Geometry: final body of the model. Coordinates: model frame, mm. A direction names the side the tool comes from. Give positions to 0.01 mm unless a question says otherwise; leave off trailing zeros. Write each loop counter-clockwise with the first axis right and the second up, starting at its lowest first coordinate (ties: lowest second). Pieces come first, ordered by that corner, then holes.
Q1. Cut plane A-A on x = -11.65. Return the cut outline in (y, z).
Q2. Line query: L1, parallel to X at y = 2.5, z = -10.5; L2, parallel to X at y = 0.5, z = -11.85; L3, parallel to X at y = 0.85, z = -11.85. Output: solid intervals per line, ascending.
Q3. Cut plane B-B on z = 4. Return the cut outline in (x, y).
Q4. Pin query (flat end, axial travel): pin 1 (1 mm diameter, centred on y = 7, z = -10.5, fed in from +X); pin 2 (0.6 mm diameter, centred on y = 1.5, z = 1.5, fed in from -X); pin 3 (3.5 mm diameter, centred on y = 7, z = 2.5, fed in from -X); pin 4 (2.5 mm diameter, centred on x = -11.65, z = -11.85, fed in from +Y) (3 decimals). Return the tip coordinate at first contact, or that it passes through.
Q5. Cut plane C-C on x = 8.5. Return the cut outline in (y, z).
Q6. Draft query along Z for faces 1 (the face through (-10.15, 0.99, -11.92)), 2 (the face through (19.213, 0.986, -19.353)), 3 (the face through (19.37, 1.01, 19.23)). Return one class per face: pulls with the +Z half, pulls with the -Z half, needs draft (parallel to the pull), parting line crosses it, or undercut.
Q7. Cut plane D-D on z = 11.85. Return the cut outline in (x, y).
Q8. Reachability of faces 4 (the face through (13.136, 6, 21)), 5 (the face through (0, 1, -9.75)), 6 (the face through (0, 4, 14)) from +Z, -Z, +X, -X, +Y, -Y: full face, straight path, thin tool, end or side. Return the list, or none.
```python
from build123d import *

# Parameters (mm, degrees)
BOSS_EXTRUDE1_DEPTH = 5
BOSS_EXTRUDE2_DEPTH = 3
CHAMFER1_SIZE       = 2
SKETCH4_R           = 1.5
SKETCH4_W           = 27.5
SKETCH4_H           = 19.5
CUT_EXTRUDE2_DEPTH  = 8
SKETCH5_W           = 28
SKETCH5_H           = 28
CUT_EXTRUDE3_DEPTH  = 3


with BuildPart() as part:
    # Sketch1 → Boss-Extrude1 (new body)
    with BuildSketch(Plane(origin=(0, 0, 0), x_dir=(1, 0, 0), z_dir=(0, 1, 0))):
        Polygon((15, 25), (25, 15), (25, -15), (15, -25), (-25, -25), (-25, 25), align=None)
    extrude(amount=BOSS_EXTRUDE1_DEPTH)

    # Sketch2 → Boss-Extrude2 (add)
    with BuildSketch(Plane(origin=(0, 5, 0), x_dir=(1, 0, 0), z_dir=(0, 1, 0))):
        Polygon((-20.5, 20.5), (-20.5, -20.5), (-22.5, -22.5), (-22.5, 22.5), align=None)
        Polygon((13.964466094, 22.5), (13.136038969, 22.5), (13.136038969, 20.5), (20.5, 13.136038969), (22.5, 13.136038969), (22.5, 13.964466094), align=None)
        Polygon((13.136038969, -20.5), (13.136038969, -22.5), (13.964466094, -22.5), (22.5, -13.964466094), (22.5, -13.136038969), (20.5, -13.136038969), align=None)
    extrude(amount=BOSS_EXTRUDE2_DEPTH)

    # Chamfer1
    chamfer1_edges = [part.edges().sort_by_distance(p)[0] for p in [
        (-5, 0, -25),
        (20, 0, -20),
        (25, 0, 0),
        (20, 0, 20),
        (-5, 0, 25),
        (-25, 0, 0),
    ]]
    chamfer(chamfer1_edges, length=CHAMFER1_SIZE)

    # Sketch4 → Cut-Extrude2 (cut)
    with BuildSketch(Plane(origin=(0, 0, 0), x_dir=(-1, 0, 0), z_dir=(0, -1, 0))):
        with Locations((-11.65, -11.85)):
            Circle(SKETCH4_R)
        with Locations((11.65, -11.85)):
            Circle(SKETCH4_R)
        with Locations((11.65, 11.85)):
            Circle(SKETCH4_R)
        with Locations((-11.65, 11.85)):
            Circle(SKETCH4_R)
        Rectangle(SKETCH4_W, SKETCH4_H)
    extrude(amount=-CUT_EXTRUDE2_DEPTH, mode=Mode.SUBTRACT)

    # Sketch5 → Cut-Extrude3 (cut)
    with BuildSketch(Plane(origin=(0, 5, 0), x_dir=(1, 0, 0), z_dir=(0, 1, 0))):
        Rectangle(SKETCH5_W, SKETCH5_H)
    extrude(amount=-CUT_EXTRUDE3_DEPTH, mode=Mode.SUBTRACT)


solid = part.part
```
Data:
1. outline: (0, -23) - (2, -25) - (5, -25) - (5, -14) - (2, -14) - (2, -13.35) - (0, -13.35) - close; (0, -10.35) - (2, -10.35) - (2, -9.75) - (0, -9.75) - close; (0, 9.75) - (2, 9.75) - (2, 10.35) - (0, 10.35) - close; (0, 13.35) - (2, 13.35) - (2, 14) - (5, 14) - (5, 25) - (2, 25) - (0, 23) - close
2. L1: x = -25 to -14, 14 to 25
2. L2: x = -23.5 to -13.15, -10.15 to 10.15, 13.15 to 23.5
2. L3: x = -23.85 to -13.15, -10.15 to 10.15, 13.15 to 23.85
3. outline: (-25, 2) - (-23, 0) - (-13.75, 0) - (-13.75, 2) - (-14, 2) - (-14, 5) - (-20.5, 5) - (-20.5, 8) - (-22.5, 8) - (-22.5, 5) - (-25, 5) - close; (13.75, 0) - (23, 0) - (25, 2) - (25, 5) - (14, 5) - (14, 2) - (13.75, 2) - close
4. pin 1: stops at x = -20.5
4. pin 2: stops at x = -24.8
4. pin 3: stops at x = -22.5
4. pin 4: passes through
5. outline: (0, -23) - (2, -25) - (5, -25) - (5, -14) - (2, -14) - (2, -9.75) - (0, -9.75) - close; (0, 9.75) - (2, 9.75) - (2, 14) - (5, 14) - (5, 25) - (2, 25) - (0, 23) - close
6. face 1: undercut
6. face 2: pulls with the -Z half
6. face 3: pulls with the +Z half
7. outline: (-25, 2) - (-23, 0) - (-13.15, 0) - (-13.15, 2) - (-14, 2) - (-14, 5) - (-20.5, 5) - (-20.5, 8) - (-22.5, 8) - (-22.5, 5) - (-25, 5) - close; (-10.15, 0) - (10.15, 0) - (10.15, 2) - (-10.15, 2) - close; (13.15, 0) - (23, 0) - (25, 2) - (25, 5) - (14, 5) - (14, 2) - (13.15, 2) - close
8. face 4: +Z, -Z, +Y
8. face 5: +Y, -Y
8. face 6: +Y
